For this review, take the finished solid that the model builds, in its own axes (mm). Face numbers are marked on the shaded views. A direction names the side the tool comes from. Round coordinates to 2 decimals unless told otherwise and drop trailing zeros. Write each loop counter-clockwise with the first axis right and the second up, starting at its lowest first coordinate (ties: lowest second). Pieces come first, ordered by that corner, then holes. Notation, with made-up numbers: M 76.25,-29 L 120.25,-29 A19 ccw 120.25,-13 Z; hole C -8,73.25 d3. An arc over 180 degrees is marked long. Use one line per item in the form item = value. Start each with the question number.
Item 1: For the marked faces 1 and 2, list the 3-axis set-ups (+Z, -Z, +X, -X, +Y, -Y) from which the entire face can be reached by the end or side of a thin tool; tool diameter is ignored.
Item 2: For line 1 (Z direction, x = 20, y = 2); line 2 (X direction, y = 0.7, z = -2.5); line 3 (Y direction, x = 5, z = -3.5), list the stretches that pass through material, from the lowest coordinate up. Write a range as [from, to].
Item 3: For P1, Ø2.5, axis at x = 21.5, z = -4, coming from the -Y side; P2, Ø4, axis at y = 0.5, z = 0, coming from the -X side; P3, Ø4, axis at x = 15, z = -2, coming from the +Y side, all flat-tipped, find the tip position at first contact; note any pin that passes through.
Item 4: Draft analysis for pull direction X (two halves, no side actions). For the marked faces 3, 4 and 5, state which applies: released by +X, released by -X, zero draft, split by the parting line, or undercut.
Item 5: Add section B-B (z = -2.5). State the section outline as (x, y) points.
Item 6: Add section A-A (y = -0.5). State the section outline as (x, z) points.
Item 7: Add section C-C (x = 4). State the section outline as (y, z) points, and give its area (3 significant figures).
Item 8: Add section D-D (y = -3.25). State the section outline as (x, z) points.
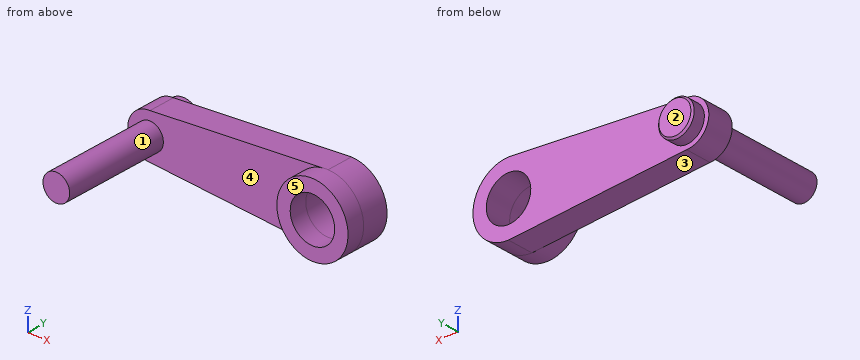
from build123d import *
from build123d.topology import SkipClean

# Parameters (mm, degrees)
SKETCH3_R           = 1.5
SKETCH3_R_2         = 2.5
BOSS_EXTRUDE1_DEPTH = 3
BOSS_EXTRUDE2_START = 2
SKETCH4_R           = 4
SKETCH4_R_2         = 2.5
BOSS_EXTRUDE2_DEPTH = 2
BOSS_EXTRUDE3_START = -15
SKETCH5_R           = 1.5
BOSS_EXTRUDE3_DEPTH = 15
SKETCH6_R           = 2
BOSS_EXTRUDE4_DEPTH = 1.5
CHAMFER1_SIZE       = 0.2


with BuildPart() as part:
    # Sketch3 → Boss-Extrude1 (new body)
    with BuildSketch(Plane(origin=(0, 0, 0), x_dir=(1, 0, 0), z_dir=(0, 1, 0))):
        with BuildLine():
            Line((0, 0), (20, -1.5))
            ThreePointArc((20, -1.5), (24, 2.5), (20, 6.5))
            Line((20, 6.5), (0, 5))
            ThreePointArc((0, 5), (-2.5, 2.5), (0, 0))
        make_face()
        with Locations(Location((0, 2.5, 0), (0, 0, 270))):
            Circle(SKETCH3_R, mode=Mode.SUBTRACT)
        with Locations(Location((20, 2.5, 0), (0, 0, 270))):
            Circle(SKETCH3_R_2, mode=Mode.SUBTRACT)
    extrude(amount=BOSS_EXTRUDE1_DEPTH)

    # Sketch4 → Boss-Extrude2 (add)
    with SkipClean():  # the faces are left unmerged after this step: merging them gives an invalid solid
        with BuildSketch(Plane.XZ.offset(BOSS_EXTRUDE2_START)):
            with Locations(Location((20, -2.5, 0), (0, 0, 270))):
                Circle(SKETCH4_R)
            with Locations(Location((20, -2.5, 0), (0, 0, 270))):
                Circle(SKETCH4_R_2, mode=Mode.SUBTRACT)
        extrude(amount=-BOSS_EXTRUDE2_DEPTH)

    # Sketch5 → Boss-Extrude3 (add)
    with SkipClean():  # the faces are left unmerged after this step: merging them gives an invalid solid
        with BuildSketch(Plane(origin=(0, 3, 0), x_dir=(1, 0, 0), z_dir=(0, 1, 0)).offset(BOSS_EXTRUDE3_START)):
            with Locations(Location((0, 2.5, 0), (0, 0, 270))):
                Circle(SKETCH5_R)
        extrude(amount=BOSS_EXTRUDE3_DEPTH)

    # Sketch6 → Boss-Extrude4 (add)
    with BuildSketch(Plane(origin=(0, 3, 0), x_dir=(1, 0, 0), z_dir=(0, 1, 0))):
        with Locations(Location((0, 2.5, 0), (0, 0, 90))):
            Circle(SKETCH6_R)
    extrude(amount=BOSS_EXTRUDE4_DEPTH)

    # Chamfer1
    chamfer1_edges = [part.edges().sort_by_distance(p)[0] for p in [
        (0, 4.5, -0.5),
    ]]
    chamfer(chamfer1_edges, length=CHAMFER1_SIZE)


solid = part.part
Calculated:
q1.face_1 = -Y
q1.face_2 = +Z, -Z, +X, -X, +Y
q2.line_1 = [-6.5, -5], [0, 1.5]
q2.line_2 = [-2.5, 17.5], [22.5, 24]
q2.line_3 = [0, 3]
q3.P1 = -2
q3.P2 = -2.45
q3.P3 = 3
q4.face_3 = released by -X
q4.face_4 = undercut
q4.face_5 = zero draft
q5.outline = M -2.5,0 L -1.5,0 L -1.5,-12 L 1.5,-12 L 1.5,0 L 16,0 L 16,-2 L 17.5,-2 L 17.5,3 L 2,3 L 2,4.3 L 1.8,4.5 L -1.8,4.5 L -2,4.3 L -2,3 L -2.5,3 Z; M 22.5,-2 L 24,-2 L 24,3 L 22.5,3 Z
q6.outline = C 0,-2.5 d3; C 20,-2.5 d8; hole C 20,-2.5 d5
q7.outline = M 0,-5.3 L 3,-5.3 L 3,0.3 L 0,0.3 Z
q7.area = 16.8 mm^2
q8.outline = C 0,-2.5 d3
